Part model, mm, in its own coordinate system. Face numbers are marked on the shaded views. Coordinates: 2 decimals unless noted, no trailing zeros. Order: outer loops, then holes, each group sorted by start corner. A loop starts at its lowest first (then second) coordinate and runs counter-clockwise, first axis right, second up.
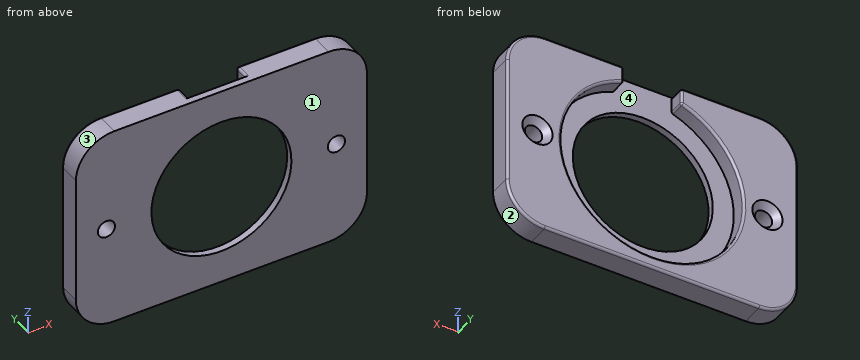
from build123d import *

# Parameters (mm, degrees)
SKETCH1_W                                       = 60.75
SKETCH1_H                                       = 43
BOSS_EXTRUDE1_DEPTH                             = 4.8
FILLET1_R                                       = 8
SKETCH2_R                                       = 19
CUT_EXTRUDE1_DEPTH                              = 3.35
SKETCH3_R                                       = 14.61
CUT_EXTRUDE2_DEPTH                              = 38.364597214
SKETCH4_W                                       = 12
SKETCH4_H                                       = 11.029070592
CUT_EXTRUDE3_DEPTH                              = 3.35
CSK_FOR_M3_FLAT_HEAD_MACHINE_SCREW1_D           = 3.6
CSK_FOR_M3_FLAT_HEAD_MACHINE_SCREW1_CSINK_D     = 6.3
CSK_FOR_M3_FLAT_HEAD_MACHINE_SCREW1_CSINK_ANGLE = 90
FILLET2_R                                       = 0.5


with BuildPart() as part:
    # Sketch1 → Boss-Extrude1 (new body)
    with BuildSketch(Plane(origin=(0, 0, 0), x_dir=(1, 0, 0), z_dir=(0, 1, 0))):
        Rectangle(SKETCH1_W, SKETCH1_H)
    extrude(amount=BOSS_EXTRUDE1_DEPTH)

    # Fillet1
    fillet1_edges = [part.edges().sort_by_distance(p)[0] for p in [
        (30.375, 2.4, 21.5),
        (-30.375, 2.4, 21.5),
        (-30.375, 2.4, -21.5),
        (30.375, 2.4, -21.5),
    ]]
    fillet(fillet1_edges, radius=FILLET1_R)

    # Sketch2 → Cut-Extrude1 (cut)
    with BuildSketch(Plane(origin=(0, 4.8, 0), x_dir=(1, 0, 0), z_dir=(0, 1, 0))):
        with Locations(Location((0, 0, 0), (0, 0, 270))):
            Circle(SKETCH2_R)
    extrude(amount=-CUT_EXTRUDE1_DEPTH, mode=Mode.SUBTRACT)

    # Sketch3 → Cut-Extrude2 (cut, through all)
    with BuildSketch(Plane(origin=(0, 1.45, 0), x_dir=(1, 0, 0), z_dir=(0, 1, 0))):
        with Locations(Location((0, 0, 0), (0, 0, 270))):
            Circle(SKETCH3_R)
    extrude(amount=-CUT_EXTRUDE2_DEPTH, mode=Mode.SUBTRACT)

    # Sketch4 → Cut-Extrude3 (cut)
    with BuildSketch(Plane(origin=(0, 4.8, 0), x_dir=(1, 0, 0), z_dir=(0, 1, 0))):
        with Locations((0, -19)):
            Rectangle(SKETCH4_W, SKETCH4_H)
    extrude(amount=-CUT_EXTRUDE3_DEPTH, mode=Mode.SUBTRACT)

    # CSK for M3 Flat Head Machine Screw1 (through all)
    with Locations(Plane(origin=(0, 4.8, 0), x_dir=(1, 0, 0), z_dir=(0, 1, 0))):
        with Locations((-24, 0), (0, 0)):
            csk_for_m3_flat_head_machine_screw1 = CounterSinkHole(CSK_FOR_M3_FLAT_HEAD_MACHINE_SCREW1_D / 2, CSK_FOR_M3_FLAT_HEAD_MACHINE_SCREW1_CSINK_D / 2, counter_sink_angle=CSK_FOR_M3_FLAT_HEAD_MACHINE_SCREW1_CSINK_ANGLE)

    # Mirror1: CSK for M3 Flat Head Machine Screw1 across plane
    add(csk_for_m3_flat_head_machine_screw1.mirror(Plane(origin=(0, 0, 0), x_dir=(0, 0, 1), z_dir=(1, 0, 0))), mode=Mode.SUBTRACT)

    # Fillet2
    fillet2_edges = [part.edges().sort_by_distance(p)[0] for p in [
        (-30.375, 4.8, 0),
        (0, 4.8, -21.5),
        (30.375, 4.8, 0),
        (-14.1875, 4.8, 21.5),
        (-28.031854249, 4.8, 19.156854249),
        (28.031854249, 4.8, 19.156854249),
        (28.031854249, 4.8, -19.156854249),
        (-28.031854249, 4.8, -19.156854249),
        (0, 4.8, -19),
        (14.1875, 4.8, 21.5),
        (6, 4.8, 19.763878189),
        (-6, 4.8, 19.763878189),
        (6, 3.125, 21.5),
        (6, 3.125, 18.027756377),
        (-6, 3.125, 21.5),
        (-6, 3.125, 18.027756377),
    ]]
    fillet(fillet2_edges, radius=FILLET2_R)


solid = part.part
Q1. Cut at B-B on z = 0. Write the cut outline in (x, y) (3 decimals).
Results list:
outline: (-30.375, 0) - (-25.8, 0) - (-25.8, 3.45) - (-27.15, 4.8) - (-29.875, 4.8) arc R0.5 ccw to (-30.375, 4.3) - close; (-22.2, 0) - (-14.61, 0) - (-14.61, 1.45) - (-19, 1.45) - (-19, 4.3) arc R0.5 ccw to (-19.5, 4.8) - (-20.85, 4.8) - (-22.2, 3.45) - close; (14.61, 0) - (22.2, 0) - (22.2, 3.45) - (20.85, 4.8) - (19.5, 4.8) arc R0.5 ccw to (19, 4.3) - (19, 1.45) - (14.61, 1.45) - close; (25.8, 0) - (30.375, 0) - (30.375, 4.3) arc R0.5 ccw to (29.875, 4.8) - (27.15, 4.8) - (25.8, 3.45) - close
Q2. Cut at A-A on x = 0. Write the cut outline in (y, z).
Results list:
outline: (0, -21.5) - (4.3, -21.5) arc R0.5 ccw to (4.8, -21) - (4.8, -19.5) arc R0.5 ccw to (4.3, -19) - (1.45, -19) - (1.45, -14.61) - (0, -14.61) - close; (0, 14.61) - (1.45, 14.61) - (1.45, 21.5) - (0, 21.5) - close
Q3. Cut at C-C on y = 2.75. Write the cut outline in (x, z) (3 decimals), and give its area (3 significant figures).
Results list:
outline: (-30.375, -13.5) arc R8 ccw to (-22.375, -21.5) - (22.375, -21.5) arc R8 ccw to (30.375, -13.5) - (30.375, 13.5) arc R8 ccw to (22.375, 21.5) - (6.5, 21.5) arc R0.5 ccw to (6, 21) - (6, 18.385) arc R0.5 ccw to (6.333, 17.913) arc R19 cw (long way) to (-6.333, 17.913) arc R0.5 ccw to (-6, 18.385) - (-6, 21) arc R0.5 ccw to (-6.5, 21.5) - (-22.375, 21.5) arc R8 ccw to (-30.375, 13.5) - close; hole circle Ø3.6 at (-24, 0); hole circle Ø3.6 at (24, 0)
area: 1,370 mm2
Q4. Pin check, flat tips, straight feed: pin 1 Ø2 at (y, z) = (2.5, 20) entering from +X; pin 2 Ø1.5 at (x, z) = (8, -12) entering from +Y; pin 3 Ø4 at (x, z) = (-24, 0) entering from +Y. Stop position of each tip, or through.
Results list:
pin 1: stops at x = 28.18
pin 2: stops at y = 1.45
pin 3: stops at y = 3.65
Q5. Wall check: line 1 along X through (y, z) = (1.35, -1.5) (3 decimals); line 2 along Y through (x, z) = (-2.5, -18); line 3 along X through (y, z) = (0.3, -2) (3 decimals). Give the ranges that are in metal, low to high.
Results list:
line 1: x = -30.375 to -24.995, -23.005 to -14.533, 14.533 to 23.005, 24.995 to 30.375
line 2: y = 0 to 1.45
line 3: x = -30.375 to -14.472, 14.472 to 30.375
Q6. Mould opens along Z. For the marked faces 1, 2, 3 and 4 say: pulls with the +Z half, pulls with the -Z half, needs draft (parallel to the pull), parting line crosses it, or undercut.
Results list:
face 1: needs draft
face 2: pulls with the -Z half
face 3: pulls with the +Z half
face 4: undercut
